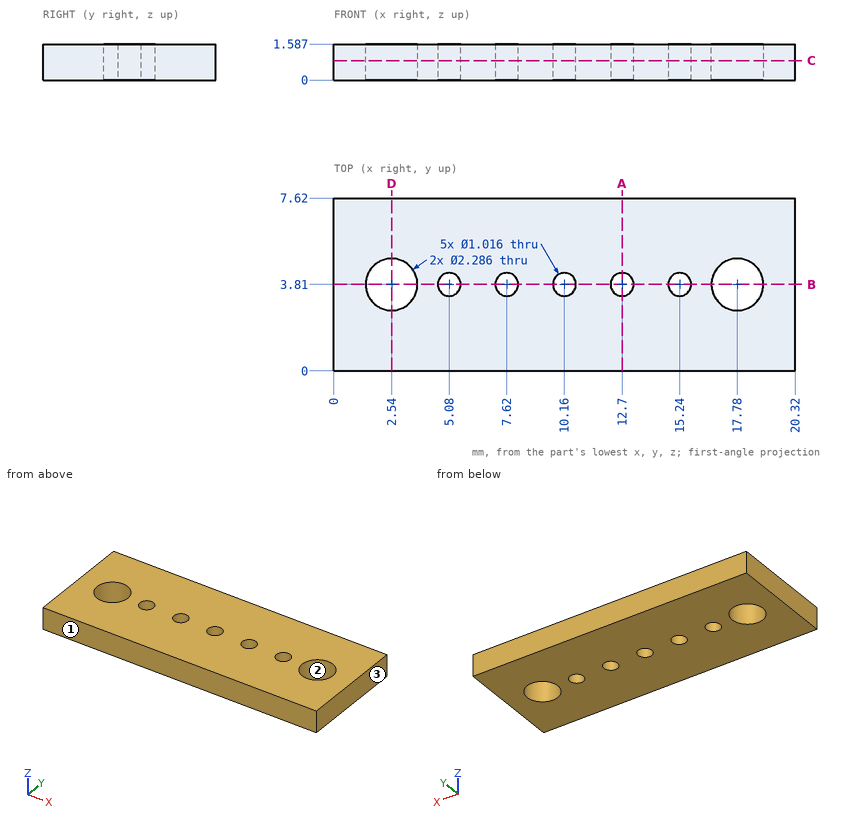
Geometry: see drawing. Coordinates: mm, zero at the bounding-box minimum. Give positions to 0.01 mm unless a question says otherwise; leave off trailing zeros. Loops run counter-clockwise (first coordinate to the right, second up) from the corner with the lowest first, then second, coordinate; pieces in that order, holes last. Notation, with made-up numbers: (-32, 30) -> (-16, 30) arc R20 ccw to (-16, 56) -> close; hole circle Ø3 at (21, -10). An arc over 180 degrees is marked (long way). Answer as a JSON object with one key per item and string values. Group by question number.
Item 1: Cut plane C-C, the plane z = 0.85. Return the cut outline in (x, y) (1 decimal).
Item 2: Pull-direction query (X, two-part tool) for the marked faces 1, 2 and 3; classes: released by +X, released by -X, zero draft, split by the parting line, or undercut.
Item 3: Line query: probe 1 along Y at (x, z) = (10.16, 0.3); probe 2 along Y at (x, z) = (2.54, 0.7); probe 3 along X at (y, z) = (4.5, 0.25). Output: solid intervals per line, ascending.
Item 4: Cut plane B-B, the plane y = 3.81. State how many separate pieces and enclosed holes the cut face has.
Item 5: Cut plane A-A, the plane x = 12.7. Return the cut outline in (y, z), and give its area (3 significant figures).
Item 6: Cut plane D-D, the plane x = 2.54. Return the cut outline in (y, z).
Checks:
{
 "1": {"outline": "(0, 0) -> (20.3, 0) -> (20.3, 7.6) -> (0, 7.6) -> close; hole circle Ø2.3 at (2.5, 3.8); hole circle Ø1 at (5.1, 3.8); hole circle Ø1 at (7.6, 3.8); hole circle Ø1 at (10.2, 3.8); hole circle Ø1 at (12.7, 3.8); hole circle Ø1 at (15.2, 3.8); hole circle Ø2.3 at (17.8, 3.8)"},
 "2": {"face 1": "zero draft", "face 2": "undercut", "face 3": "released by +X"},
 "3": {"probe 1": "y = 0 to 3.3, 4.32 to 7.62", "probe 2": "y = 0 to 2.67, 4.95 to 7.62", "probe 3": "x = 0 to 1.63, 3.45 to 16.87, 18.69 to 20.32"},
 "4": {"separate pieces": "8", "enclosed holes": "0"},
 "5": {"outline": "(0, 0) -> (3.3, 0) -> (3.3, 1.59) -> (0, 1.59) -> close; (4.32, 0) -> (7.62, 0) -> (7.62, 1.59) -> (4.32, 1.59) -> close", "area": "10.5 mm²"},
 "6": {"outline": "(0, 0) -> (2.67, 0) -> (2.67, 1.59) -> (0, 1.59) -> close; (4.95, 0) -> (7.62, 0) -> (7.62, 1.59) -> (4.95, 1.59) -> close"}
}
